from build123d import *

# Parameters (mm, degrees)
ESBO_O1_R                = 3
RESSALTO_EXTRUS_O1_DEPTH = 60
ESBO_O2_R                = 5
RESSALTO_EXTRUS_O2_DEPTH = 6
FILETE1_R                = 0.5
CORTE_EXTRUS_O1_DEPTH    = 3
CHANFRO3_SIZE            = 0.5
CHANFRO4_SIZE            = 0.5


with BuildPart() as part:
    # Esboço1 → Ressalto-extrusão1 (new body)
    with BuildSketch(Plane(origin=(0, 0, 0), x_dir=(1, 0, 0), z_dir=(0, 1, 0))):
        with Locations(Location((0, 0, 0), (0, 0, 270))):
            Circle(ESBO_O1_R)
    extrude(amount=-RESSALTO_EXTRUS_O1_DEPTH)

    # Esboço2 → Ressalto-extrusão2 (add)
    with BuildSketch(Plane(origin=(0, 0, 0), x_dir=(1, 0, 0), z_dir=(0, 1, 0))):
        with Locations(Location((0, 0, 0), (0, 0, 270))):
            Circle(ESBO_O2_R)
    extrude(amount=RESSALTO_EXTRUS_O2_DEPTH)

    # Filete1
    filete1_edges = [part.edges().sort_by_distance(p)[0] for p in [
        (0, 6, -5),
    ]]
    fillet(filete1_edges, radius=FILETE1_R)

    # Esboço3 → Corte-extrusão1 (cut)
    with BuildSketch(Plane(origin=(0, 6, 0), x_dir=(1, 0, 0), z_dir=(0, 1, 0))):
        Polygon((2.886751346, 0), (1.443375673, 2.5), (-1.443375673, 2.5), (-2.886751346, 0), (-1.443375673, -2.5), (1.443375673, -2.5), align=None)
    extrude(amount=-CORTE_EXTRUS_O1_DEPTH, mode=Mode.SUBTRACT)

    # Chanfro3
    chanfro3_edges = [part.edges().sort_by_distance(p)[0] for p in [
        (2.165063509, 6, 1.25),
        (2.165063509, 6, -1.25),
        (0, 6, -2.5),
        (-2.165063509, 6, -1.25),
        (-2.165063509, 6, 1.25),
        (0, 6, 2.5),
    ]]
    chamfer(chanfro3_edges, length=CHANFRO3_SIZE)

    # Chanfro4
    chanfro4_edges = [part.edges().sort_by_distance(p)[0] for p in [
        (0, -60, -3),
    ]]
    chamfer(chanfro4_edges, length=CHANFRO4_SIZE)


solid = part.part
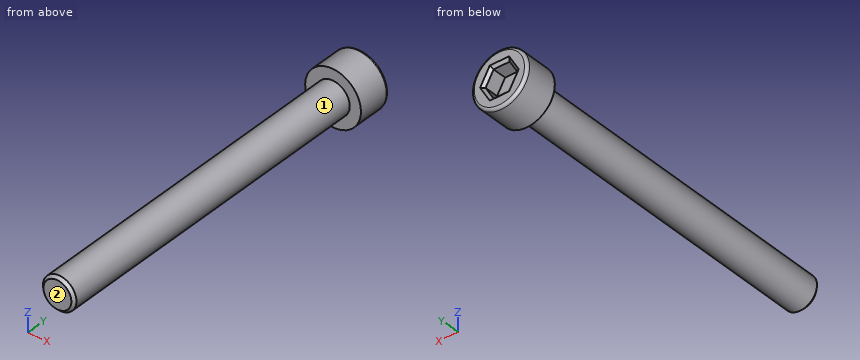
For this review, take the finished solid that the model builds, in its own axes (mm). Face numbers are marked on the shaded views. A direction names the side the tool comes from. Give positions to 0.01 mm unless a question says otherwise; leave off trailing zeros. Order: outer loops, then holes, each group sorted by start corner. A loop starts at its lowest first (then second) coordinate and runs counter-clockwise, first axis right, second up. Notation, with made-up numbers: M 29.5,61.5 L 67.5,61.5 A26 cw 67.5,98.5 Z; hole C 15.25,47.25 d4. An arc over 180 degrees is marked long. Answer in a Markdown table with one row per item. Add a question column.
(1) For the marked faces 1 and 2, list the 3-axis set-ups (+Z, -Z, +X, -X, +Y, -Y) from which the entire face can be reached by the end or side of a thin tool; tool diameter is ignored.
(2) Consider section A-A on y = -23.5. State the section outline as (x, z) points, and give its area (3 significant figures).
(3) For pin 1 (2.5 mm diameter, centred on x = 0, z = -1, fed in from +Y); pin 2 (6 mm diameter, centred on x = 2, y = -18, fed in from +Z); pin 3 (5 mm diameter, centred on x = -3.5, z = -3, fed in from +Y); pin 4 (6 mm diameter, centred on y = -27, z = -1, fed in from +X), all flat-tipped, find the tip position at first contact; note any pin that passes through.
(4) Wall thickness on probe 1 along Y at (x, z) = (-2.5, -3.5); probe 2 along X at (y, z) = (-2, 0); probe 3 along Y at (x, z) = (0.25, 0.75): over which ranges is each line inside the solid? List them lowest first. Write a range as [from, to].
Evaluation:
| question | item | result |
|---|---|---|
| 1 | face 1 | -Y |
| 1 | face 2 | +Z, -Z, +X, -X, -Y |
| 2 | outline | C 0,0 d6 |
| 2 | area | 28.3 mm^2 |
| 3 | pin 1 | stops at y = 3 |
| 3 | pin 2 | stops at z = 3 |
| 3 | pin 3 | stops at y = 6 |
| 3 | pin 4 | stops at x = 3 |
| 4 | probe 1 | y = [0, 6] |
| 4 | probe 2 | x = [-3, 3] |
| 4 | probe 3 | y = [-60, 3] |
